from build123d import *

# Parameters (mm, degrees)
PAD020_DEPTH            = 18
SKETCH034_W             = 12.810354
SKETCH034_H             = 8.636197
POCKET003_DEPTH         = 10
HOLE007_D               = 3.4
HOLE007_DEPTH           = 25
HOLE007_CBORE_D         = 6.1
HOLE007_CBORE_DEPTH     = 3.4
SKETCH037_R             = 1.7
HOLE008_DEPTH           = 25
CHAMFER001_SIZE         = 1
BODY020_PLACEMENT_ANGLE = 180


with BuildPart() as part:
    # Sketch033 → Pad020 (new body)
    with BuildSketch(Plane.XZ):
        with BuildLine():
            ThreePointArc((-5, 0), (0, -5), (5, 0))
            Line((5, 0), (5, 7.200889))
            Line((-5, 7.200889), (5, 7.200889))
            Line((-5, 7.200889), (-5, 0))
        make_face()
    extrude(amount=PAD020_DEPTH)

    # Sketch034 (on Face5 of Pad020) → Pocket003 (cut)
    with BuildSketch(Plane(origin=(0, 0, 0), x_dir=(1, 0, 0), z_dir=(0, 1, 0))):
        with Locations((-0.681749, 1.0732765)):
            Rectangle(SKETCH034_W, SKETCH034_H)
    extrude(amount=-POCKET003_DEPTH, mode=Mode.SUBTRACT)

    # Hole007
    with Locations(Plane(origin=(0, -10, 0), x_dir=(1, 0, 0), z_dir=(0, 1, 0))):
        with Locations((-0.07012, 0.834162)):
            CounterBoreHole(HOLE007_D / 2, HOLE007_CBORE_D / 2, HOLE007_CBORE_DEPTH, depth=HOLE007_DEPTH)

    # Sketch037 (on Face6 of Hole007) → Hole008 (cut)
    with BuildSketch(Plane(origin=(0, 0, 3.244822), x_dir=(1, 0, 0), z_dir=(0, 0, -1))):
        with Locations((0, 6.488995)):
            Circle(SKETCH037_R)
    extrude(amount=-HOLE008_DEPTH, mode=Mode.SUBTRACT)

    # Chamfer001
    chamfer001_edges = [part.edges().sort_by_distance(p)[0] for p in [
        (0, -10, 3.244822),
    ]]
    chamfer(chamfer001_edges, length=CHAMFER001_SIZE)


with BuildPart() as part_1:
    # Body020 placement: moved
    add(part.part.moved(Location((24, 66.5, 19))).rotate(Axis((24, 66.5, 19), (0, 1, 0)), BODY020_PLACEMENT_ANGLE))


solid = part_1.part
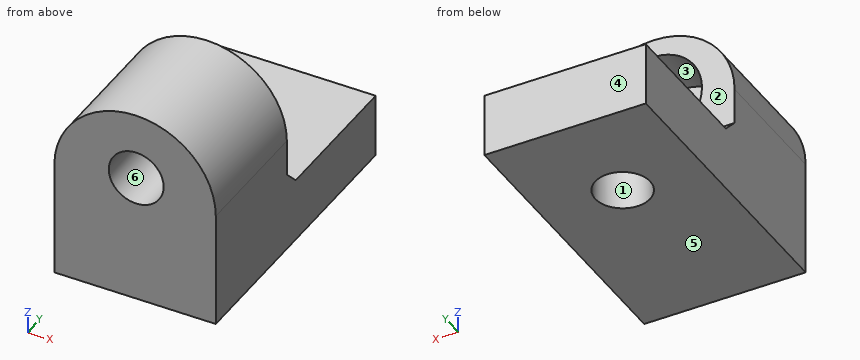
The model under review builds one solid part; all positions refer to its coordinate system, in mm. Face numbers are marked on the shaded views. A direction names the side the tool comes from. Round coordinates to 2 decimals unless told otherwise and drop trailing zeros. Write each loop counter-clockwise with the first axis right and the second up, starting at its lowest first coordinate (ties: lowest second). Pieces come first, ordered by that corner, then holes. Notation, with made-up numbers: (37.25, 87) - (58.25, 87) arc R11 ccw to (58.25, 106) - close; hole circle Ø3 at (49, -23.5). An arc over 180 degrees is marked (long way). One line per item, written item: value. Start each with the question number.
1. To check wall thickness, follow L1, parallel to Y at x = 26.25, z = 21.5; L2, parallel to Z at x = 28.5, y = 64.5; L3, parallel to X at y = 59.75, z = 14.75. State the ranges of each line that lie inside material, in increasing order. Write a range as from..to.
2. The part is to be moulded in two halves that separate along Z. For the marked faces 4, 5 and 6, say which applies: released by +Z, released by -Z, zero draft, split by the parting line, or undercut.
3. Consider section D-D on z = 13. Write out the cut boundary in (x, y), and give its area (3 significant figures).
4. Clearance check with flat-ended pins moving along their axes: P1, Ø1.8, axis at x = 23.5, z = 20.5, coming from the +Y side; P2, Ø6, axis at x = 23, z = 20.5, coming from the +Y side; P3, Ø1.5, axis at y = 56, z = 22, coming from the -X side. State where each tip first meets the part, or that it passes through.
5. Consider section C-C on x = 20. Write out the cut boundary in (y, z), and give its area (3 significant figures).
6. Machinability: for the marked faces 1, 2 and 3, which of the approach directions +Z, -Z, +X, -X, +Y, -Y give a long, thin tool a straight path to every point of the face, cutting with its end or side? Answer none if there is none.
7. Consider section B-B on y = 54. Write out the cut boundary in (x, z), and give its area (3 significant figures).
8. Consider section A-A on x = 25.5. Write out the cut boundary in (y, z).
Checks:
1. L1: y = 48.5..53.1
1. L2: z = 11.8..15.76
1. L3: x = 19..22.32, 25.68..29
2. face 4: zero draft
2. face 5: released by -Z
2. face 6: undercut
3. outline: (19, 48.5) - (29, 48.5) - (29, 66.5) - (19, 66.5) - close; hole circle Ø3.4 at (24, 60.01)
3. area: 171 mm^2
4. P1: stops at y = 53.1
4. P2: stops at y = 56.5
4. P3: stops at x = 19.53
5. outline: (48.5, 11.8) - (66.5, 11.8) - (66.5, 15.76) - (57.5, 15.76) - (56.5, 16.76) - (56.5, 22) - (48.5, 22) - close
5. area: 122 mm^2
6. face 1: +Z, -Z
6. face 2: +Z, +X, -X, +Y
6. face 3: +Y
7. outline: (19, 11.8) - (29, 11.8) - (29, 19) arc R5 ccw to (19, 19) - close; hole circle Ø6.1 at (24.07, 19.83)
7. area: 82.1 mm^2
8. outline: (48.5, 11.8) - (59.21, 11.8) - (59.21, 15.76) - (57.5, 15.76) - (56.5, 16.76) - (56.5, 17.14) - (53.1, 17.14) - (53.1, 18.91) - (48.5, 18.91) - close; (48.5, 20.75) - (53.1, 20.75) - (53.1, 22.53) - (56.5, 22.53) - (56.5, 23.77) - (48.5, 23.77) - close; (60.81, 11.8) - (66.5, 11.8) - (66.5, 15.76) - (60.81, 15.76) - close
